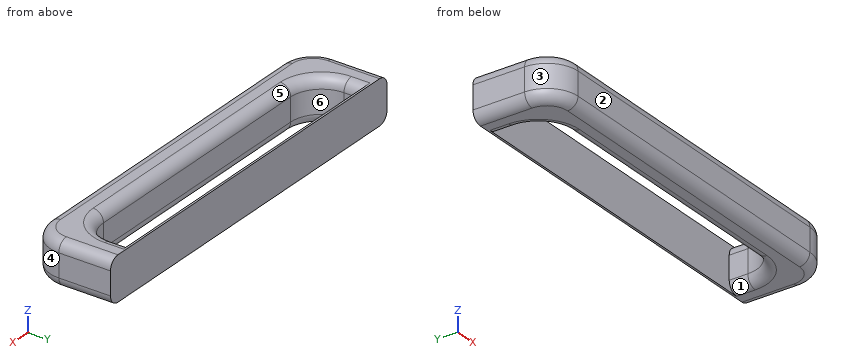
from build123d import *

# Parameters (mm, degrees)
SKETCH008_W     = 185.746766
SKETCH008_H     = 21.2714
PAD006_DEPTH    = 40
SKETCH009_W     = 155.746766
SKETCH009_H     = 24
POCKET002_DEPTH = 21.2724
FILLET_R        = 15
FILLET001_R     = 5


with BuildPart() as part:
    # Sketch008 (on Face1 of CopyPocket001) → Pad006 (new body)
    with BuildSketch(Plane.XZ.offset(825)):
        with Locations((0, -79.507206)):
            Rectangle(SKETCH008_W, SKETCH008_H)
    extrude(amount=PAD006_DEPTH)

    # Sketch009 (on Face4 of Pad006) → Pocket002 (cut, through all)
    with BuildSketch(Plane(origin=(0, 0, -68.871506), x_dir=(-1, 0, 0), z_dir=(0, 0, 1))):
        with Locations((0, 838)):
            Rectangle(SKETCH009_W, SKETCH009_H)
    extrude(amount=-POCKET002_DEPTH, mode=Mode.SUBTRACT)

    # Fillet
    fillet_edges = [part.edges().sort_by_distance(p)[0] for p in [
        (77.873383, -850, -79.507206),
        (-77.873383, -850, -79.507206),
        (-92.873383, -865, -79.507206),
        (92.873383, -865, -79.507206),
    ]]
    fillet(fillet_edges, radius=FILLET_R)

    # Fillet001
    fillet001_edges = [part.edges().sort_by_distance(p)[0] for p in [
        (0, -865, -68.871506),
        (0, -865, -90.142906),
        (0, -850, -68.871506),
        (0, -850, -90.142906),
    ]]
    fillet(fillet001_edges, radius=FILLET001_R)


solid = part.part
The listing builds one solid part. Answer for the finished solid, in the listing's coordinates (mm). Face numbers are marked on the shaded views. A direction names the side the tool comes from. Round coordinates to 2 decimals unless told otherwise and drop trailing zeros. Order: outer loops, then holes, each group sorted by start corner. A loop starts at its lowest first (then second) coordinate and runs counter-clockwise, first axis right, second up. Notation, with made-up numbers: M 73,3.5 L 124,3.5 A23 cw 124,22.5 Z; hole C 57.5,75 d3. An arc over 180 degrees is marked long. Answer in a Markdown table with one row per item. Add a question column.
1) Which of the six approach directions +Z, -Z, +X, -X, +Y, -Y give full straight-line access (tool end or side, diameter ignored) to the marked faces 4, 5 and 6?
2) Determine the mould class of the marked faces 1, 2 and 3 for opening direction X: pulls with the +X half, pulls with the -X half, needs draft (parallel to the pull), parting line crosses it, or undercut.
3) Consider line 1 along Y through (x, z) = (62, -83.75); line 2 along X through (y, z) = (-831, -77.5); line 3 along Y through (x, z) = (55, -86.5). Determine where each line is inside the solid, lowest interval first. Write a range as from..to.
4) The part is cut by section B-B on x = 6. Determine the outline of the cut face in (y, z).
5) The part is cut by section C-C on y = -830.5. Determine the outline of the cut face in (x, z), plus the area to 3 significant figures.
6) The part is cut by section A-A on z = -78. Determine the outline of the cut face in (x, y), plus the area to 3 significant figures.
Findings below:
| question | item | result |
|---|---|---|
| 1 | face 4 | +Z, -Z, +X, -Y |
| 1 | face 5 | +Z |
| 1 | face 6 | +Z, -Z |
| 2 | face 1 | undercut |
| 2 | face 2 | needs draft |
| 2 | face 3 | pulls with the -X half |
| 3 | line 1 | y = -865..-850, -826..-825 |
| 3 | line 2 | x = -92.87..-77.87, 77.87..92.87 |
| 3 | line 3 | y = -864.81..-850.19, -826..-825 |
| 4 | outline | M -865,-85.14 A5 ccw -860,-90.14 L -855,-90.14 A5 ccw -850,-85.14 L -850,-73.87 A5 ccw -855,-68.87 L -860,-68.87 A5 ccw -865,-73.87 Z; M -826,-90.14 L -825,-90.14 L -825,-68.87 L -826,-68.87 Z |
| 5 | outline | M -92.87,-85.14 A5 ccw -87.87,-90.14 L -82.87,-90.14 A5 ccw -77.87,-85.14 L -77.87,-73.87 A5 ccw -82.87,-68.87 L -87.87,-68.87 A5 ccw -92.87,-73.87 Z; M 77.87,-85.14 A5 ccw 82.87,-90.14 L 87.87,-90.14 A5 ccw 92.87,-85.14 L 92.87,-73.87 A5 ccw 87.87,-68.87 L 82.87,-68.87 A5 ccw 77.87,-73.87 Z |
| 5 | area | 595 mm² |
| 6 | outline | M -92.87,-850 A15 ccw -77.87,-865 L 77.87,-865 A15 ccw 92.87,-850 L 92.87,-825 L -92.87,-825 Z; hole M -77.87,-835 A15 ccw -62.87,-850 L 62.87,-850 A15 ccw 77.87,-835 L 77.87,-826 L -77.87,-826 Z |
| 6 | area | 3,690 mm² |
